For this review, use the dimensioned drawing (mm, ordinates from the lowest corner) and the shaded views. A direction names the side the tool comes from. Round coordinates to 2 decimals unless told otherwise and drop trailing zeros. Write each loop counter-clockwise with the first axis right and the second up, starting at its lowest first coordinate (ties: lowest second). Pieces come first, ordered by that corner, then holes. Notation, with made-up numbers: M 61,-16.75 L 67,-16.75 A10 cw 67,2.25 Z; hole C 72,60 d10. An arc over 180 degrees is marked long. Write each question's results on one line, items separated by ' | '. Start each with the question number.
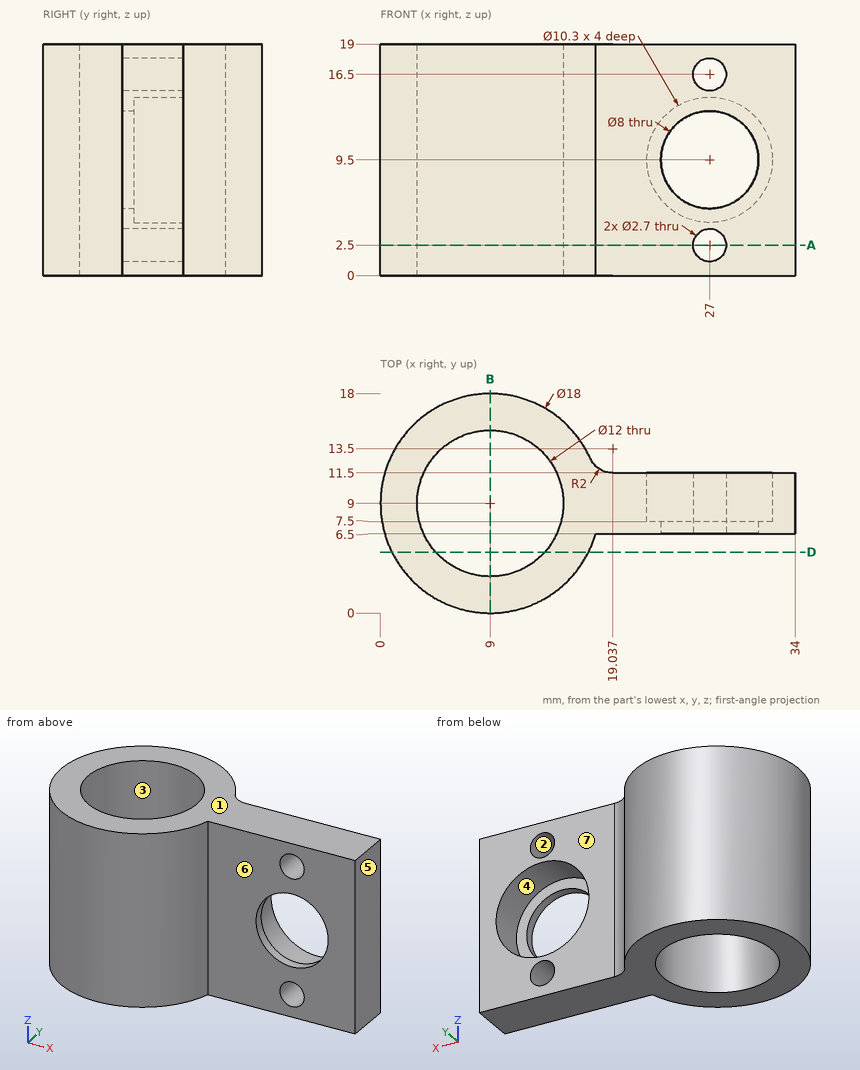
Item 1: Insertion check: P1, Ø8, axis at x = 24.5, z = 8.5, coming from the +Y side; P2, Ø3, axis at x = 12.5, z = 6.5, coming from the -Y side (1 decimal); P3, Ø5, axis at x = 25, z = 8.5, coming from the +Y side. Each pin has a flat end and moves straight along its axis. Give the tip position at first contact, or say it passes through.
Item 2: We need section B-B on x = 9. State the section outline as (y, z) points, then the cut area to 3 significant figures.
Item 3: For probe 1 along Z at (x, y) = (27, 9.5); probe 2 along Z at (x, y) = (27, 6.85); probe 3 along X at (y, z) = (10.5, 6.5) (1 decimal), list the stretches that pass through material, from the lowest coordinate up.
Item 4: For the marked faces 5, 6 and 7, list the 3-axis set-ups (+Z, -Z, +X, -X, +Y, -Y) from which the entire face can be reached by the end or side of a thin tool; tool diameter is ignored.
Item 5: Mouldability with a two-part tool opening along Z and no side actions: class the marked faces 1, 2, 3 and 4 as pulls with the +Z half, pulls with the -Z half, needs draft (parallel to the pull), parting line crosses it, or undercut.
Item 6: We need section D-D on y = 5. State the section outline as (x, z) points.
Item 7: We need section A-A on z = 2.5. State how many separate pieces and enclosed holes the cut face has, then the cut area to 3 significant figures.
Numbers:
1) P1: stops at y = 11.5 | P2: stops at y = 0.2 | P3: stops at y = 7.5
2) outline: M 0,0 L 3,0 L 3,19 L 0,19 Z; M 15,0 L 18,0 L 18,19 L 15,19 Z | area: 114 mm^2
3) probe 1: z = 0 to 1.15, 3.85 to 4.35, 14.65 to 15.15, 17.85 to 19 | probe 2: z = 0 to 1.15, 3.85 to 5.5, 13.5 to 15.15, 17.85 to 19 | probe 3: x = 0.1 to 3.2, 14.8 to 22.8, 31.2 to 34
4) face 5: +Z, -Z, +X, +Y, -Y | face 6: +Z, -Z, +X, -Y | face 7: +Z, -Z, +X, +Y
5) face 1: pulls with the +Z half | face 2: undercut | face 3: needs draft | face 4: undercut
6) outline: M 0.94,0 L 4.53,0 L 4.53,19 L 0.94,19 Z; M 13.47,0 L 17.06,0 L 17.06,19 L 13.47,19 Z
7) separate pieces: 2 | enclosed holes: 1 | area: 209 mm^2
